from build123d import *

# Parameters (mm, degrees)
SKETCH_1_R          = 12.5
EXTRUDE_1_DEPTH     = 49.8
SKETCH_2_R          = 3.5
EXTRUDE_2_DEPTH     = 2.5
SKETCH_3_R          = 2
EXTRUDE_3_DEPTH     = 11.5
CUT_EXTRUDE_START   = -9
CUT_EXTRUDE_1_DEPTH = 9
SKETCH_5_R          = 1.5
CUT_EXTRUDE_2_DEPTH = 3
SKETCH_6_R          = 4
EXTRUDE_4_DEPTH     = 8


with BuildPart() as part:
    # 草图1 → 凸台-拉伸1 (new body)
    with BuildSketch(Plane.XY):
        Circle(SKETCH_1_R)
    extrude(amount=EXTRUDE_1_DEPTH)

    # 草图2 → 凸台-拉伸2 (add)
    with BuildSketch(Plane(origin=(0, 0, 0), x_dir=(-1, 0, 0), z_dir=(0, 0, -1))):
        Circle(SKETCH_2_R)
    extrude(amount=EXTRUDE_2_DEPTH)

    # 草图3 → 凸台-拉伸3 (add)
    with BuildSketch(Plane(origin=(0, 0, -2.5), x_dir=(-1, 0, 0), z_dir=(0, 0, -1))):
        Circle(SKETCH_3_R)
    extrude(amount=EXTRUDE_3_DEPTH)

    # 草图4 → 切除-拉伸1 (cut)
    with BuildSketch(Plane(origin=(0, 0, -14), x_dir=(-1, 0, 0), z_dir=(0, 0, -1)).offset(CUT_EXTRUDE_START)):
        with BuildLine():
            Line((-1.322875656, 1.5), (0, 1.5))
            Line((0, 1.5), (1.322875656, 1.5))
            ThreePointArc((1.322875656, 1.5), (0, 2), (-1.322875656, 1.5))
        make_face()
    extrude(amount=CUT_EXTRUDE_1_DEPTH, mode=Mode.SUBTRACT)

    # 草图5 → 切除-拉伸2 (cut)
    with BuildSketch(Plane(origin=(0, 0, 0), x_dir=(-1, 0, 0), z_dir=(0, 0, -1))):
        with Locations((8.5, 0)):
            Circle(SKETCH_5_R)
        with Locations(Location((-8.5, 0, 0), (0, 0, 180))):
            Circle(SKETCH_5_R)
    extrude(amount=-CUT_EXTRUDE_2_DEPTH, mode=Mode.SUBTRACT)

    # 草图6 → 凸台-拉伸4 (add)
    with BuildSketch(Plane.XY.offset(49.8)):
        Circle(SKETCH_6_R)
    extrude(amount=EXTRUDE_4_DEPTH)


solid = part.part
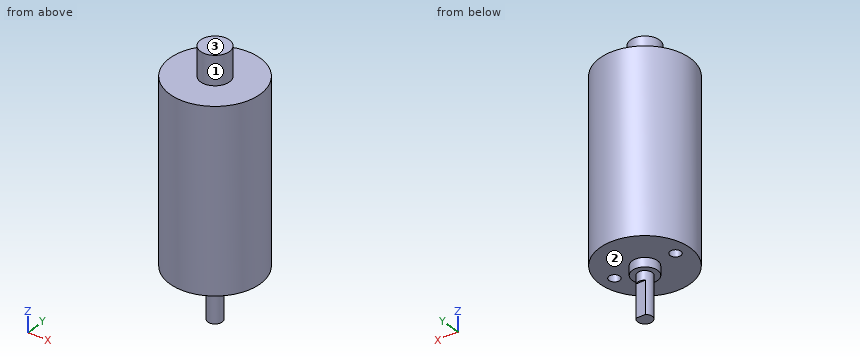
Input: part model. Units: mm. Frame: model coordinates. Face numbers are marked on the shaded views. A direction names the side the tool comes from. Give positions to 0.01 mm unless a question says otherwise; leave off trailing zeros. Order: outer loops, then holes, each group sorted by start corner. A loop starts at its lowest first (then second) coordinate and runs counter-clockwise, first axis right, second up. Notation, with made-up numbers: M 60,36 L 102,36 A24 cw 102,52 Z; hole C 41,83.25 d10. An arc over 180 degrees is marked long. Answer as a JSON object with one key per item and string values.
1. Ray query, line 1 (Z direction, x = 3.5, y = -0.75); line 2 (Y direction, x = 8.5, z = 2.2); line 3 (Z direction, x = 1.25, y = -9.75). Return the intervals inside material, ascending. Write a range as [from, to].
Result sheet:
{"line 1": "[0, 57.8]", "line 2": "[-9.17, -1.5], [1.5, 9.17]", "line 3": "[0, 49.8]"}
2. Cut plane B-B, the plane x = 0. Output: boundary loops of the cut face in (y, z), and give its area (3 significant figures).
Result sheet:
{"outline": "M -12.5,0 L -3.5,0 L -3.5,-2.5 L -2,-2.5 L -2,-14 L 1.5,-14 L 1.5,-5 L 2,-5 L 2,-2.5 L 3.5,-2.5 L 3.5,0 L 12.5,0 L 12.5,49.8 L 4,49.8 L 4,57.8 L -4,57.8 L -4,49.8 L -12.5,49.8 Z", "area": "1,370 mm²"}
3. Cut plane D-D, the plane x = -8.5. Output: boundary loops of the cut face in (y, z), and give its area (3 significant figures).
Result sheet:
{"outline": "M -9.17,0 L -1.5,0 L -1.5,3 L 1.5,3 L 1.5,0 L 9.17,0 L 9.17,49.8 L -9.17,49.8 Z", "area": "904 mm²"}
4. First-contact query: P1, Ø2.5, axis at x = 9, y = 0.5, coming from the -Z side; P2, Ø2, axis at x = -5.5, z = 19, coming from the -Y side; P3, Ø4, axis at y = 6, z = 42.5, coming from the -X side. Flat tips, straight axial feed; report the tip coordinate or a pass-through.
Result sheet:
{"P1": "z = 0", "P2": "y = -11.66", "P3": "x = -11.84"}
5. Cut plane C-C, the plane z = 36. Output: boundary loops of the cut face in (x, y).
Result sheet:
{"outline": "C 0,0 d25"}
6. Cut plane A-A, the plane y = 0. Output: boundary loops of the cut face in (x, z).
Result sheet:
{"outline": "M -12.5,0 L -10,0 L -10,3 L -7,3 L -7,0 L -3.5,0 L -3.5,-2.5 L -2,-2.5 L -2,-14 L 2,-14 L 2,-2.5 L 3.5,-2.5 L 3.5,0 L 7,0 L 7,3 L 10,3 L 10,0 L 12.5,0 L 12.5,49.8 L 4,49.8 L 4,57.8 L -4,57.8 L -4,49.8 L -12.5,49.8 Z"}
7. Reachability of the marked faces 1, 2 and 3 from +Z, -Z, +X, -X, +Y, -Y: full face, straight path, thin tool, end or side. Return the list, or none.
Result sheet:
{"face 1": "+Z", "face 2": "-Z", "face 3": "+Z, +X, -X, +Y, -Y"}
